Geometry: see drawing. Coordinates: mm, zero at the bounding-box minimum. Give positions to 0.01 mm unless a question says otherwise; leave off trailing zeros. Write each loop counter-clockwise with the first axis right and the second up, starting at its lowest first coordinate (ties: lowest second). Pieces come first, ordered by that corner, then holes. Notation, with made-up numbers: M 86.5,33 L 129.5,33 A12 cw 129.5,49 Z; hole C 30.25,-0.5 d1. An arc over 180 degrees is marked long. Use one line per item in the form item = value. Start each with the question number.
Item 1: Section query D-D on x = 1.5. Return loops of the section in (y, z), then the cut area to 3 significant figures.
Item 2: Material intervals for line 1 along X through (y, z) = (20.5, 6.25) (1 decimal); line 2 along Z through (x, y) = (7.25, 36.5); line 3 along Z through (x, y) = (9.75, 8) (1 decimal), sorted ascending. Write a range as from..to.
Item 3: Section query B-B on z = 11.5. Return loops of the section in (x, y) (1 decimal).
Item 4: Section query A-A on x = 6.75. Return loops of the section in (y, z) (1 decimal), then the cut area to 3 significant figures.
Item 5: Contact query for flat-ended pins moving along their axis: P1, Ø2, axis at y = 17, z = 2.5, coming from the -X side; P2, Ø8, axis at x = 3, y = 15, coming from the +Z side; P3, Ø1.5, axis at y = 10.5, z = 7.5, coming from the -X side; P4, Ø1, axis at x = 3, y = 8, coming from the +Z side (1 decimal). Output: stop coordinate, or through.
Item 6: Pull-direction query (Z, two-part tool) for the marked faces 1, 2 and 3; classes: released by +Z, released by -Z, zero draft, split by the parting line, or undercut.
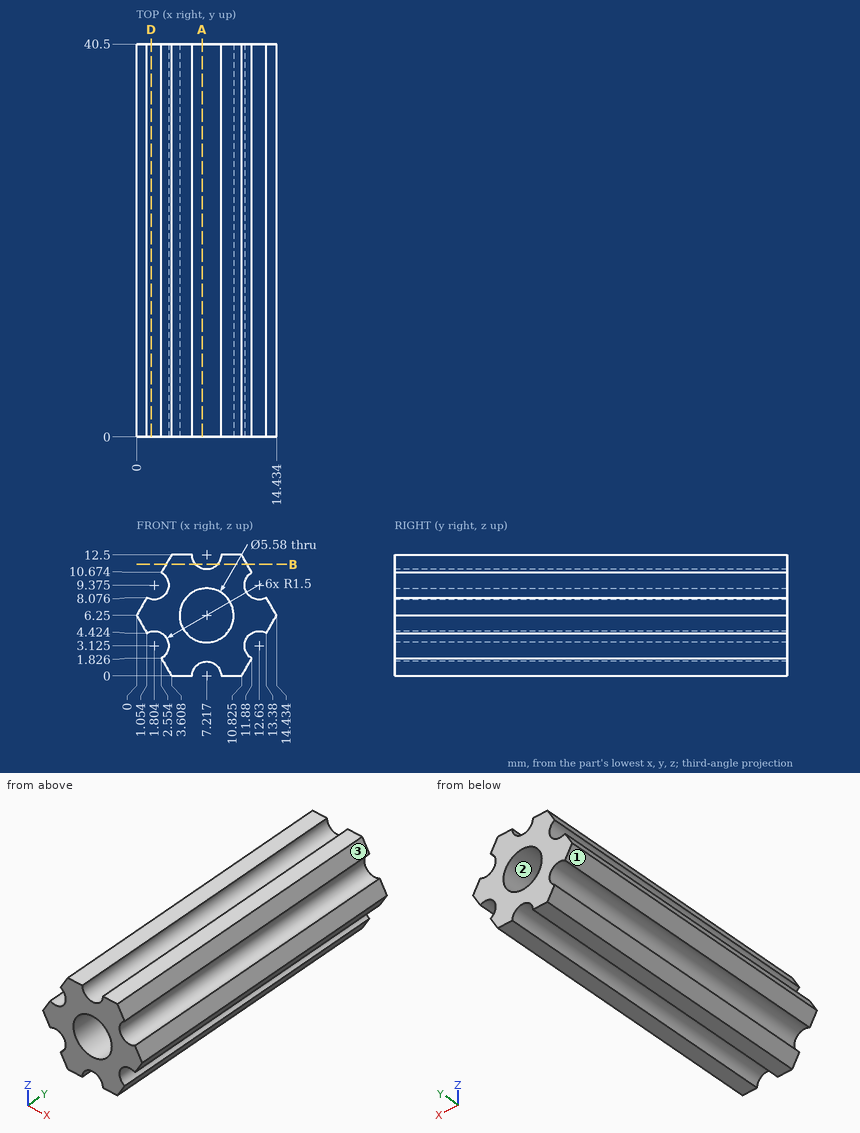
Answer sheet:
q1.outline = M 0,4.59 L 40.5,4.59 L 40.5,7.91 L 0,7.91 Z
q1.area = 134 mm2
q2.line_1 = 0..4.4, 10..14.4
q2.line_2 = 1.5..3.46, 9.04..11
q2.line_3 = 0..5.1, 7.4..12.5
q3.outline = M 3,0 L 6.1,0 L 6.1,40.5 L 3,40.5 Z; M 8.3,0 L 11.4,0 L 11.4,40.5 L 8.3,40.5 Z
q4.outline = M 0,1.4 L 40.5,1.4 L 40.5,3.5 L 0,3.5 Z; M 0,9 L 40.5,9 L 40.5,11.1 L 0,11.1 Z
q4.area = 168 mm2
q5.P1 = 2.55
q5.P2 = 12.5
q5.P3 = 0.29
q5.P4 = 12.3
q6.face_1 = released by -Z
q6.face_2 = undercut
q6.face_3 = released by +Z
